Work out the finished part from the listing and answer in its coordinate system (mm). A direction names the side the tool comes from. Round coordinates to 2 decimals unless told otherwise and drop trailing zeros. Write each loop counter-clockwise with the first axis right and the second up, starting at its lowest first coordinate (ties: lowest second). Pieces come first, ordered by that corner, then holes. Notation, with made-up numbers: (35.25, 82.25) - (47.25, 82.25) arc R22 cw to (47.25, 103.25) - close; hole circle Ø7 at (4.25, 44.25). An arc over 180 degrees is marked (long way). Write item = value, one per line. Start each with the question number.
from build123d import *

# Parameters (mm, degrees)
SKETCH_1_R          = 12.4
EXTRUDE_1_DEPTH     = 63
SKETCH_2_R          = 3.5
EXTRUDE_2_DEPTH     = 4
EXTRUDE_3_DEPTH     = 8
SKETCH_4_R          = 1.5
CUT_EXTRUDE_1_DEPTH = 10


with BuildPart() as part:
    # 草图1 → 凸台-拉伸1 (new body)
    with BuildSketch(Plane.XY):
        Circle(SKETCH_1_R)
    extrude(amount=EXTRUDE_1_DEPTH)

    # 草图2 → 凸台-拉伸2 (add)
    with BuildSketch(Plane.XY.offset(63)):
        Circle(SKETCH_2_R)
    extrude(amount=EXTRUDE_2_DEPTH)

    # 草图3 → 凸台-拉伸3 (add)
    with BuildSketch(Plane.XY.offset(67)):
        with BuildLine():
            Line((-1.41, 1.418414608), (-1.41, -1.418414608))
            ThreePointArc((-1.41, -1.418414608), (2, 0), (-1.41, 1.418414608))
        make_face()
    extrude(amount=EXTRUDE_3_DEPTH)

    # 草图4 → 切除-拉伸1 (cut)
    with BuildSketch(Plane.XY.offset(63)):
        with Locations((0, -8.5)):
            Circle(SKETCH_4_R)
        with Locations((0, 8.5)):
            Circle(SKETCH_4_R)
    extrude(amount=-CUT_EXTRUDE_1_DEPTH, mode=Mode.SUBTRACT)


solid = part.part
1. Which of the six approach directions +Z, -Z, +X, -X, +Y, -Y give full straight-line access (tool end or side, diameter ignored) to faces 5 (the face through (0, 0, 0)), 6 (the face through (0, -10, 58)), 7 (the face through (-1.41, 0, 71))?
2. Find section B-B on z = 68. Give the vertices of the cut face in (x, y).
3. Find section D-D on z = 36.5. Give the vertices of the cut face in (x, y).
4. Find section C-C on x = 6.5. Give the vertices of the cut face in (y, z), plus the area to 3 significant figures.
5. Each of these flat-tipped pins is pushed along its axis until it touches: pin 1 (5 mm diameter, centred on y = -9.5, z = 30, fed in from +X); pin 2 (3.5 mm diameter, centred on x = 0.5, y = -8.5, fed in from +Z); pin 3 (1 mm diameter, centred on y = 7, z = 13.5, fed in from -X). Where does it stop, or does it pass through?
6. Find section A-A on y = 0. Give the vertices of the cut face in (x, z).
7. For a pull along X with two mould halves and no side action, classify faces 1 (the face through (0, 7, 58)), 2 (the face through (-2, 0, 67)), 3 (the face through (0, 9, 53)), 4 (the face through (2, 0, 71)) as released by +X, released by -X, zero draft, split by the parting line, or undercut.
8. Consider line 1 (Z direction, x = -9.25, y = 7.75); line 2 (Z direction, x = 0.5, y = 7.75); line 3 (X direction, y = 0.25, z = 17). Determine where each line is inside the solid, lowest interval first.
Answer key:
q1.face_5 = -Z, +X, -X, +Y, -Y
q1.face_6 = +Z
q1.face_7 = +Z, -X, +Y, -Y
q2.outline = (-1.41, -1.42) arc R2 ccw (long way) to (-1.41, 1.42) - close
q3.outline = circle Ø24.8 at (0, 0)
q4.outline = (-10.56, 0) - (10.56, 0) - (10.56, 63) - (-10.56, 63) - close
q4.area = 1,330 mm²
q5.pin_1 = 10.24
q5.pin_2 = 63
q5.pin_3 = -10.56
q6.outline = (-12.4, 0) - (12.4, 0) - (12.4, 63) - (3.5, 63) - (3.5, 67) - (2, 67) - (2, 75) - (-1.41, 75) - (-1.41, 67) - (-3.5, 67) - (-3.5, 63) - (-12.4, 63) - close
q7.face_1 = undercut
q7.face_2 = zero draft
q7.face_3 = undercut
q7.face_4 = split by the parting line
q8.line_1 = 0 to 63
q8.line_2 = 0 to 53
q8.line_3 = -12.4 to 12.4
